Build history of the part. All positions in model axes, mm. A direction names the side the tool comes from. Round coordinates to 2 decimals unless told otherwise and drop trailing zeros. Write each loop counter-clockwise with the first axis right and the second up, starting at its lowest first coordinate (ties: lowest second). Pieces come first, ordered by that corner, then holes. Notation, with made-up numbers: (27, 40.5) - (31, 40.5) arc R20 ccw to (31, 75.5) - close; hole circle Ø7 at (69.5, -36). An arc over 180 degrees is marked (long way). Answer as a JSON object with one key per item and string values. Group by question number.
Item 1: Two-plate mould, pull along Y, no slides. Class faces 4 (the flat face through (2, -1, -1)), 5 (the cylindrical face through (1.11, 0.08, 1.9)), 6 (the flat face through (0.5, 0.75, 0)): +Y half, -Y half, draft (parallel to the pull), parting line (faces both ways), or undercut.
Item 2: Probe line 1 (Z direction, x = 7, y = -0.9); line 2 (X direction, y = 1.25, z = 0.05); line 3 (Z direction, x = 19.5, y = 0.65). List the from-to ranges inside material, lowest first. Write a range as from..to.
Item 3: Slice it at A-A, the plane x = 7.25. List the corners of the cut face in (y, z).
Item 4: Which spindle directions (+Z, -Z, +X, -X, +Y, -Y) get a long thin tool onto all of the face, cutting with end or side? Do faces 1 (the flat face through (0, 1, 0)), 2 (the flat face through (0.5, -0.75, 0)), 3 (the cylindrical face through (12, -1, 0)). Say none if no direction does.
Item 5: Flat gauge pin, fed straight in: pin 1 (2 mm diameter, centred on x = 11.5, y = 1, fed in from +Z). Where does the tip first touch, or does it go through?
from build123d import *

# Parameters (mm, degrees)
SKETCH1_R           = 1.9
BASEHEAD_DEPTH      = 2
SKETCH2_R           = 1
BASEBODY_DEPTH      = 20
HEXAGONSOCKET_DEPTH = 1
TOPFILLET_R         = 0.25
CHAMFER1_SIZE       = 0.1


with BuildPart() as part:
    # Sketch1 → BaseHead (new body)
    with BuildSketch(Plane(origin=(0, 0, 0), x_dir=(0, 0, -1), z_dir=(1, 0, 0))):
        Circle(SKETCH1_R)
    extrude(amount=BASEHEAD_DEPTH)

    # Sketch2 → BaseBody (add)
    with BuildSketch(Plane(origin=(2, 0, 0), x_dir=(0, 0, -1), z_dir=(1, 0, 0))):
        Circle(SKETCH2_R)
    extrude(amount=BASEBODY_DEPTH)

    # Sketch3 → HexagonSocket (cut)
    with BuildSketch(Plane(origin=(0, 0, 0), x_dir=(0, 0, -1), z_dir=(1, 0, 0))):
        Polygon((0.866025404, 0), (0.433012702, 0.75), (-0.433012702, 0.75), (-0.866025404, 0), (-0.433012702, -0.75), (0.433012702, -0.75), align=None)
    extrude(amount=HEXAGONSOCKET_DEPTH, mode=Mode.SUBTRACT)

    # Sketch4 → Cut-Revolve1 (revolve, cut)
    with BuildSketch(Plane(origin=(-4.19613823, 0.75, 0), x_dir=(-1, 0, 0), z_dir=(0, 0, 1))):
        Polygon((-5.19613823, 1.5), (-5.629150931, 0.75), (-5.19613823, 0.75), align=None)
    revolve(axis=Axis((0.838992387, 0, 0), (-1, 0, 0)), mode=Mode.SUBTRACT)

    # TopFillet
    topfillet_edges = [part.edges().sort_by_distance(p)[0] for p in [
        (0, 0, 1.9),
    ]]
    fillet(topfillet_edges, radius=TOPFILLET_R)

    # Chamfer1
    chamfer1_edges = [part.edges().sort_by_distance(p)[0] for p in [
        (22, 0, 1),
    ]]
    chamfer(chamfer1_edges, length=CHAMFER1_SIZE)


solid = part.part
Geometry says:
{
 "1": {"face 4": "draft", "face 5": "parting line", "face 6": "undercut"},
 "2": {"line 1": "z = -0.44..0.44", "line 2": "x = 0..2", "line 3": "z = -0.76..0.76"},
 "3": {"outline": "circle Ø2 at (0, 0)"},
 "4": {"face 1": "+Z, -Z, -X, +Y, -Y", "face 2": "-X", "face 3": "+X"},
 "5": {"pin 1": "stops at z = 1"}
}
